Model file for the job. Use its own axes, mm. A direction names the side the tool comes from. Coordinates: 2 decimals unless noted, no trailing zeros. Loops run counter-clockwise (first coordinate to the right, second up) from the corner with the lowest first, then second, coordinate; pieces in that order, holes last. Notation, with made-up numbers: M -40,35 L 2,35 A10 cw 2,51 Z; hole C 26,41 d6. An arc over 180 degrees is marked long. One line per question, with ' | ' between items. Start each with the question number.
```python
from build123d import *

# Parameters (mm, degrees)
F0_W     = 10
F0_H     = 5
F1_DEPTH = 10
F2_W     = 3
F2_H     = 5
F3_DEPTH = 4
F4_W     = 10
F4_H     = 5
F5_DEPTH = 1.1
F6_R     = 0.5
F7_R     = 0.5
F8_SIZE  = 1
F10_D    = 1.75
F12_D    = 1.75
F14_D    = 2


with BuildPart() as f1:
    # F0 (on Top) → F1 (new body)
    with BuildSketch(Plane.XY):
        Rectangle(F0_W, F0_H)
    extrude(amount=F1_DEPTH)

    # F2 (on face) → F3 (cut)
    with BuildSketch(Plane(origin=(0, 2.5, 0), x_dir=(-1, 0, 0), z_dir=(0, 1, 0))):
        with Locations((0, 2.5)):
            Rectangle(F2_W, F2_H)
    extrude(amount=-F3_DEPTH, mode=Mode.SUBTRACT)

    # F4 (on face) → F5 (cut)
    with BuildSketch(Plane(origin=(0, 2.5, 0), x_dir=(-1, 0, 0), z_dir=(0, 1, 0))):
        with Locations((0, 2.5)):
            Rectangle(F4_W, F4_H)
    extrude(amount=-F5_DEPTH, mode=Mode.SUBTRACT)

    # F6
    f6_edges = [f1.edges().sort_by_distance(p)[0] for p in [
        (1.5, -1.5, 2.5),
        (-1.5, -1.5, 2.5),
        (0, -1.5, 5),
    ]]
    fillet(f6_edges, radius=F6_R)

    # F7
    f7_edges = [f1.edges().sort_by_distance(p)[0] for p in [
        (-3.25, 1.4, 5),
        (3.25, 1.4, 5),
    ]]
    fillet(f7_edges, radius=F7_R)

    # F8
    f8_edges = [f1.edges().sort_by_distance(p)[0] for p in [
        (5, -2.5, 5),
        (-5, -2.5, 5),
    ]]
    chamfer(f8_edges, length=F8_SIZE)

    # F10 (through all)
    with Locations(Plane(origin=(0, 1.4, 0), x_dir=(-1, 0, 0), z_dir=(0, 1, 0))):
        with Locations((-3.2, 2), (3.2, 2)):
            Hole(F10_D / 2)

    # F12 (through all)
    with Locations(Plane(origin=(-5, 0, 0), x_dir=(0, -1, 0), z_dir=(-1, 0, 0))):
        with Locations((0, 7.5)):
            Hole(F12_D / 2)

    # F14 (through all)
    with Locations(Plane.XY.offset(10)):
        with Locations((0, 0)):
            Hole(F14_D / 2)


solid = f1.part
```
(1) Drill centre lines: line 1 (Y direction, x = 3.9, z = 7.5) (3 decimals); line 2 (Z direction, x = -2.5, y = -0.6) (3 decimals); line 3 (Z direction, x = 3.2, y = -1.35) (3 decimals). Where is each one in solid material? Low to high. Write a range as [from, to].
(2) Band-saw the part on A-A on x = -3.2. Write the cut outline in (y, z) (3 decimals), then the cut area to 3 significant figures.
(3) 3-axis set-ups, long thin cutter, end or side, ignore diameter. For faces 1 (the face through (1.5, 0, 2)), 2 (the face through (2.774, -0.874, 7.538)), 3 (the face through (4, 1.4, 3)): which of +Z, -Z, +X, -X, +Y, -Y reach the whole face in a straight line?
(4) Pin check, flat tips, straight feed: P1, Ø3, axis at x = -3.2, z = 2, coming from the +Y side; P2, Ø0.6, axis at x = 0, z = 2.5, coming from the +Y side. Stop position of each tip, or through.
(5) Band-saw the part on B-B on y = -0.5. Write the cut outline in (x, z) (3 decimals).
(6) Band-saw the part on C-C on z = 7.5. Write the cut outline in (x, y) (3 decimals), then the cut area to 3 significant figures.
(7) Band-saw the part on D-D on z = 2.5. Write the cut outline in (x, y), then the cut area to 3 significant figures.
(8) Two-plate mould, pull along Y, no slides. Class faces 4 (the face through (-2.71, 0.835, 7.763)), 5 (the face through (-4, 1.4, 3)), 6 (the face through (-0.07, 1.15, 10)): pulls with the +Y half, pulls with the -Y half, needs draft (parallel to the pull), parting line crosses it, or undercut.
Computed values:
1) line 1: [-2.5, -0.875], [0.875, 2.5] | line 2: [0, 1.475], [2.525, 6.863], [8.137, 10] | line 3: [0, 1.125], [2.875, 10]
2) outline: M -2.5,0 L 1.4,0 L 1.4,1.125 L -2.5,1.125 Z; M -2.5,2.875 L 1.4,2.875 L 1.4,4.5 A0.5 cw 1.9,5 L 2.5,5 L 2.5,10 L -2.5,10 Z; hole C 0,7.5 d1.75 | area: 35.3 mm^2
3) face 1: -Z, +Y | face 2: +X, -X | face 3: -Z, +X, -X, +Y
4) P1: y = 1.4 | P2: y = -1.5
5) outline: M -5,0 L -1.5,0 L -1.5,5 L -0.866,5 L -0.866,6.782 L -5,6.782 Z; M -5,8.218 L -0.866,8.218 L -0.866,10 L -5,10 Z; M 0.866,5 L 1.5,5 L 1.5,0 L 5,0 L 5,6.782 L 0.866,6.782 Z; M 0.866,8.218 L 5,8.218 L 5,10 L 0.866,10 Z; hole C -3.2,2 d1.75; hole C 3.2,2 d1.75
6) outline: M -5,-1.5 L -4,-2.5 L 4,-2.5 L 5,-1.5 L 5,-0.875 L 0.484,-0.875 A1 cw -0.484,-0.875 L -5,-0.875 Z; M -5,0.875 L -0.484,0.875 A1 cw 0.484,0.875 L 5,0.875 L 5,2.5 L -5,2.5 Z | area: 31.3 mm^2
7) outline: M -5,-1.5 L -4,-2.5 L -3.92,-2.5 L -3.92,1.4 L -5,1.4 Z; M -2.48,-2.5 L 2.48,-2.5 L 2.48,1.4 L 1.5,1.4 L 1.5,-1 A0.5 cw 1,-1.5 L -1,-1.5 A0.5 cw -1.5,-1 L -1.5,1.4 L -2.48,1.4 Z; M 3.92,-2.5 L 4,-2.5 L 5,-1.5 L 5,1.4 L 3.92,1.4 Z | area: 18.2 mm^2
8) face 4: undercut | face 5: pulls with the +Y half | face 6: needs draft
